For this review, take the finished solid that the model builds, in its own axes (mm). A direction names the side the tool comes from. Coordinates: 2 decimals unless noted, no trailing zeros. Loops run counter-clockwise (first coordinate to the right, second up) from the corner with the lowest first, then second, coordinate; pieces in that order, holes last. Notation, with made-up numbers: M 59.25,-16 L 85.25,-16 A15 ccw 85.25,-5 Z; hole C 56.5,-39.75 d4. An arc over 180 degrees is marked long. Write item = value, one per line.
from build123d import *

# Parameters (mm, degrees)
BASPROSKE_W         = 4
BASPROSKE_H         = 7.875
TOOTHCUT_DEPTH      = 12.833480046
TEETHCUTS_COUNT     = 12
TEETHCUTS_ANGLE     = 330
BORSKE_R            = 1
BORE_DEPTH          = 50.0000508
SKETCH1_R           = 3.125
SKETCH1_R_2         = 2.125
BOSS_EXTRUDE1_DEPTH = 2
SKETCH2_R           = 2
CUT_EXTRUDE1_DEPTH  = 3


with BuildPart() as part:
    # BasProSke → Base-Revolve (revolve)
    with BuildSketch(Plane(origin=(0, 0, 0), x_dir=(1, 0, 0), z_dir=(0, 1, 0)), mode=Mode.PRIVATE) as base_revolve_sk:
        with Locations((2, 3.9375)):
            Rectangle(BASPROSKE_W, BASPROSKE_H)
    revolve(base_revolve_sk.sketch.rotate(Axis((-10, 0, 0), (1, 0, 0)), 180), axis=Axis((-10, 0, 0), (1, 0, 0)))

    # TooCutSke → ToothCut (cut, through all)
    with BuildSketch(Plane(origin=(0, 0, 0), x_dir=(0, 0, -1), z_dir=(1, 0, 0))):
        with BuildLine():
            ThreePointArc((0.631439839, 5.305305014), (0, 5.34275), (-0.631439839, 5.305305014))
            ThreePointArc((-0.631439839, 5.305305014), (-0.93992237, 6.654932089), (-1.876748184, 7.674251521))
            ThreePointArc((-1.876748184, 7.674251521), (0, 7.9004), (1.876748184, 7.674251521))
            ThreePointArc((1.876748184, 7.674251521), (0.93992237, 6.654932089), (0.631439839, 5.305305014))
        make_face()
    toothcut = extrude(amount=TOOTHCUT_DEPTH, mode=Mode.SUBTRACT)

    # TeethCuts: ToothCut ×12 about axis
    teethcuts_axis = Axis((-10, 0, 0), (1, 0, 0))
    for i in range(1, TEETHCUTS_COUNT):
        add(toothcut.rotate(teethcuts_axis, i * TEETHCUTS_ANGLE / (TEETHCUTS_COUNT - 1)), mode=Mode.SUBTRACT)

    # BorSke → Bore (cut, symmetric)
    with BuildSketch(Plane(origin=(0, 0, 0), x_dir=(0, 0, -1), z_dir=(1, 0, 0))):
        with Locations(Location((0, 0, 0), (0, 0, 180))):
            Circle(BORSKE_R)
    extrude(amount=BORE_DEPTH, both=True, mode=Mode.SUBTRACT)

    # Sketch1 → Boss-Extrude1 (add)
    with BuildSketch(Plane.ZY):
        with Locations(Location((0, 0, 0), (0, 0, 180))):
            Circle(SKETCH1_R)
        Circle(SKETCH1_R_2, mode=Mode.SUBTRACT)
    extrude(amount=BOSS_EXTRUDE1_DEPTH)

    # Sketch2 → Cut-Extrude1 (cut)
    with BuildSketch(Plane(origin=(4, 0, 0), x_dir=(0, 0, -1), z_dir=(1, 0, 0))):
        Circle(SKETCH2_R)
    extrude(amount=-CUT_EXTRUDE1_DEPTH, mode=Mode.SUBTRACT)


solid = part.part
Q1. Add section C-C (y = -6). Write out the cut boundary in (x, z), and give its area (3 significant figures).
Solved:
outline = M 0,-2.49 L 4,-2.49 L 4,-0.7 L 0,-0.7 Z; M 0,0.7 L 4,0.7 L 4,2.49 L 0,2.49 Z
area = 14.4 mm²
Q2. For pin 1 Ø1.6 at (y, z) = (0, 0) entering from -X; pin 2 Ø2.5 at (y, z) = (0, 0) entering from -X, all flat-tipped, find the tip position at first contact; note any pin that passes through.
Solved:
pin_1 = through
pin_2 = 0
Q3. Add section A-A (z = 0). Write out the cut boundary in (x, y) (3 decimals), and give its area (3 significant figures).
Solved:
outline = M -2,-3.125 L 0,-3.125 L 0,-5.343 L 4,-5.343 L 4,-2 L 1,-2 L 1,-1 L 0,-1 L 0,-2.125 L -2,-2.125 Z; M -2,2.125 L 0,2.125 L 0,1 L 1,1 L 1,2 L 4,2 L 4,5.343 L 0,5.343 L 0,3.125 L -2,3.125 Z
area = 32.7 mm²
Q4. For line 1 along Y through (x, z) = (0.6, 0); line 2 along Y through (x, z) = (3.35, 0); line 3 along Z through (x, y) = (1.2, 5.5), list the stretches that pass through material, from the lowest coordinate up.
Solved:
line_1 = -5.34 to -1, 1 to 5.34
line_2 = -5.34 to -2, 2 to 5.34
line_3 = -5.64 to -4.54, -2.38 to -0.63, 0.63 to 2.38, 4.54 to 5.64
Q5. Machinability: for faces 1 (the face through (0.507, 0.976, -0.217)), 2 (the face through (1, -1, -1)), which of the approach directions +Z, -Z, +X, -X, +Y, -Y give a long, thin tool a straight path to every point of the face, cutting with its end or side? Answer none if there is none.
Solved:
face_1 = +X, -X
face_2 = +X
Q6. Add section D-D (z = -4). Write out the cut boundary in (x, y), and give its area (3 significant figures).
Solved:
outline = M 0,-5.2 L 4,-5.2 L 4,5.2 L 0,5.2 Z
area = 41.6 mm²
